Geometry: see drawing. Coordinates: mm, zero at the bounding-box minimum. Coordinates: 2 decimals unless noted, no trailing zeros. Write each loop counter-clockwise with the first axis right and the second up, starting at its lowest first coordinate (ties: lowest second). Pieces come first, ordered by that corner, then holes. Notation, with made-up numbers: M 7.25,1.5 L 25.25,1.5 A7 cw 25.25,5.5 Z; hole C -11.75,48 d5. An arc over 180 degrees is marked long. One line per item, written item: value. Start each with the question number.
Item 1: Pin query (flat end, axial travel): P1, Ø3, axis at x = 11, z = 64.5, coming from the +Y side; P2, Ø10, axis at y = 114.5, z = 64, coming from the -X side. Return the tip coordinate at first contact, or that it passes through.
Item 2: Cut plane A-A, the plane y = 63. Output: boundary loops of the cut face in (x, z) (1 decimal).
Item 3: Cut plane B-B, the plane z = 55. Output: boundary loops of the cut face in (x, y) (1 decimal).
Item 4: Ray query, L1, parallel to Z at x = 4, y = 34.5 (1 decimal); L2, parallel to X at y = 145.5, z = 22 (1 decimal). Return the intervals inside material, ascending. Write a range as from..to.
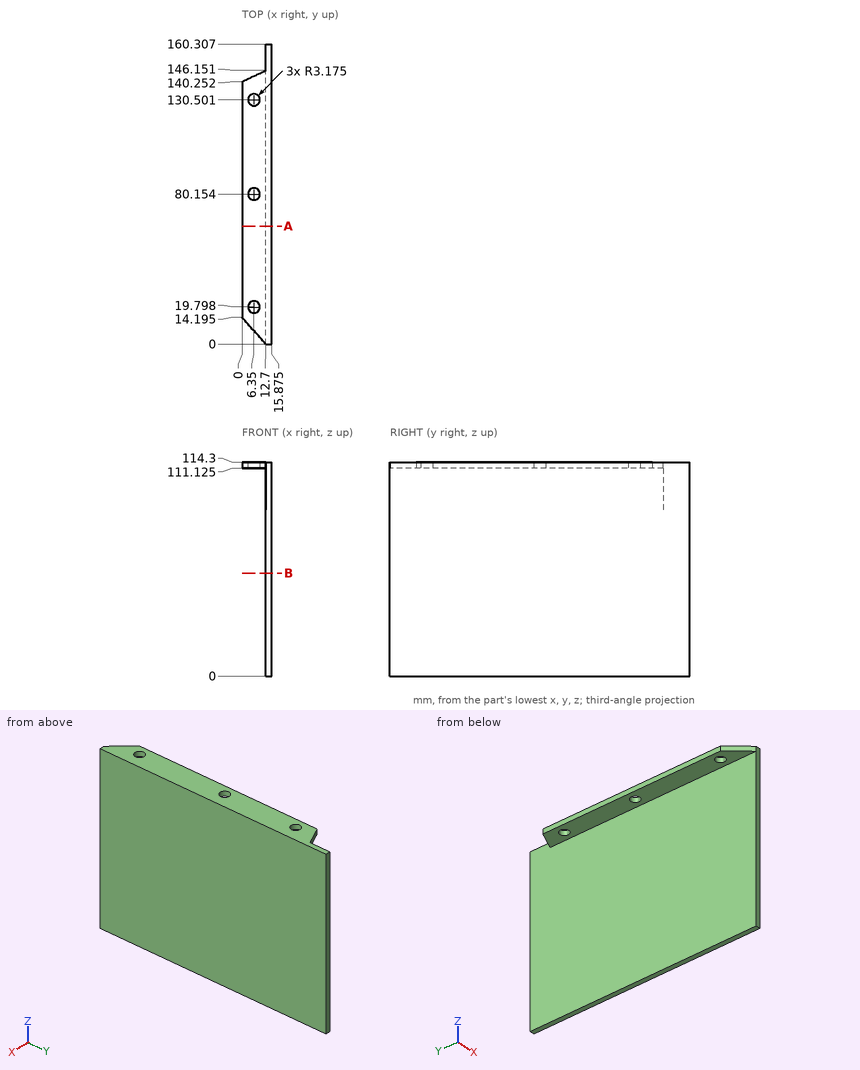
From the geometry:
1. P1: passes through
1. P2: stops at x = 12.7
2. outline: M 0,111.1 L 12.7,111.1 L 12.7,0 L 15.9,0 L 15.9,114.3 L 0,114.3 Z
3. outline: M 12.7,0 L 15.9,0 L 15.9,160.3 L 12.7,160.3 Z
4. L1: z = 111.1..114.3
4. L2: x = 12.7..15.9
